Part print with two shaded views. Sizes in mm from the minimum x, y, z corner. A direction names the side the tool comes from. Give positions to 0.01 mm unless a question says otherwise; leave off trailing zeros. Order: outer loops, then holes, each group sorted by start corner. A loop starts at its lowest first (then second) coordinate and runs counter-clockwise, first axis right, second up. Notation, with made-up numbers: M 22.25,77 L 26.25,77 A10 ccw 26.25,90 Z; hole C -3,-24 d7. An arc over 180 degrees is marked long. Return JSON: item names as keys, results as strings. Group by question number.
1. Slice it at A-A on z = 14. List the corners of the cut face in (x, y).
2. Pin check, flat tips, straight feed: pin 1 (4 mm diameter, centred on y = 15.5, z = 14.5, fed in from +X); pin 2 (6 mm diameter, centred on x = 16, y = 5, fed in from +Z). Stop position of each tip, or through.
3. 3-axis set-ups, long thin cutter, end or side, ignore diameter. For the marked faces 1 and 2: which of +Z, -Z, +X, -X, +Y, -Y reach the whole face in a straight line?
4. Slice it at B-B on y = 9. Give the number of separate pieces and of enclosed holes in the cut face, then the cut area to 3 significant figures.
5. Two-plate mould, pull along Z, no slides. Class the marked faces 3, 4 and 5: released by +Z, released by -Z, zero draft, split by the parting line, or undercut.
6. Slice it at C-C on x = 14. List the corners of the cut face in (y, z), then the cut area to 3 significant figures.
7. Wall check: probe 1 along Y at (x, z) = (1.75, 14); probe 2 along Z at (x, y) = (13, 12.5). Give the ranges that are in metal, low to high. Write a range as [from, to].
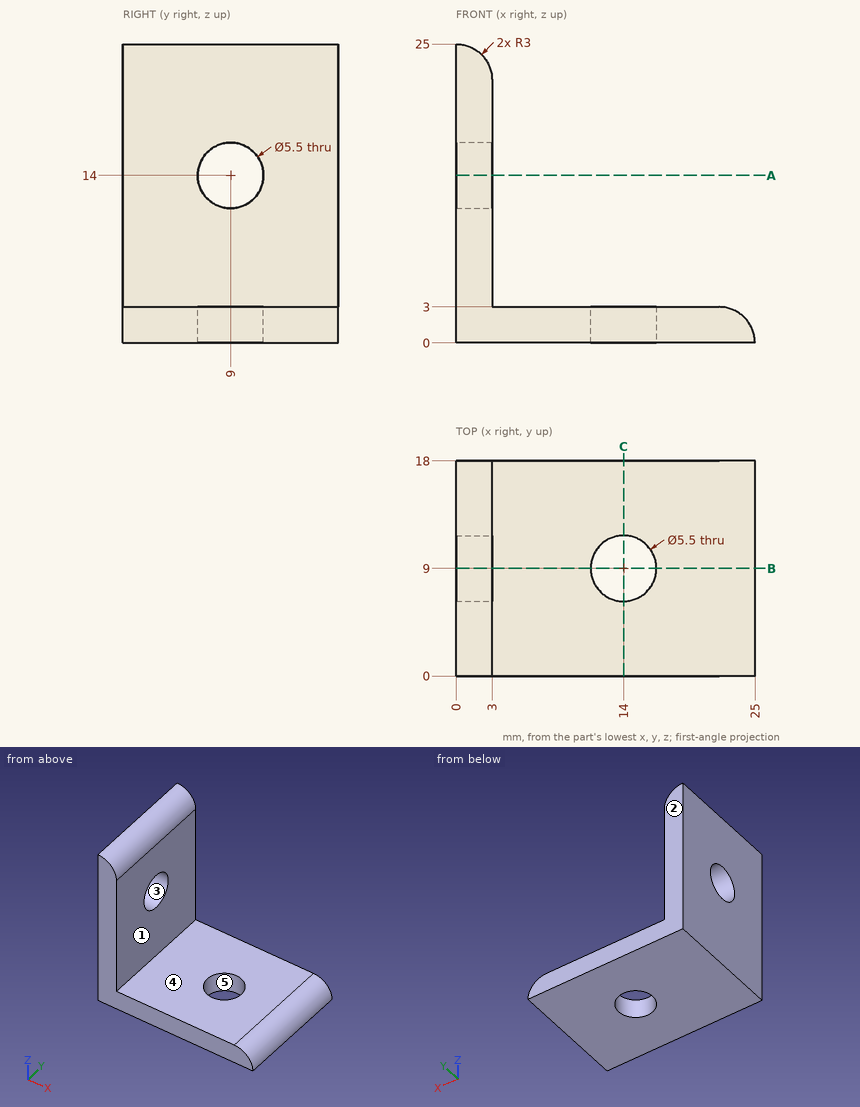
Result:
{
 "1": {"outline": "M 0,0 L 3,0 L 3,6.25 L 0,6.25 Z; M 0,11.75 L 3,11.75 L 3,18 L 0,18 Z"},
 "2": {"pin 1": "stops at x = 3", "pin 2": "stops at z = 3"},
 "3": {"face 1": "+Z, +X, +Y, -Y", "face 2": "+Z, -Z, +X, -X, +Y"},
 "4": {"separate pieces": "3", "enclosed holes": "0", "area": "104 mm2"},
 "5": {"face 3": "undercut", "face 4": "released by +Z", "face 5": "zero draft"},
 "6": {"outline": "M 0,0 L 6.25,0 L 6.25,3 L 0,3 Z; M 11.75,0 L 18,0 L 18,3 L 11.75,3 Z", "area": "37.5 mm2"},
 "7": {"probe 1": "y = [0, 6.25], [11.75, 18]", "probe 2": "z = [0, 3]"}
}
